Geometry: final body of the model. Coordinates: model frame, mm. Coordinates: 2 decimals unless noted, no trailing zeros. Loops run counter-clockwise (first coordinate to the right, second up) from the corner with the lowest first, then second, coordinate; pieces in that order, holes last. Notation, with made-up numbers: (55.5, 10.25) - (114.5, 10.25) arc R35 ccw to (114.5, 45.25) - close; hole circle Ø1 at (-14.5, 81). An arc over 180 degrees is marked (long way). Write each question's results on one line, items separated by ' | '. Start each with the question number.
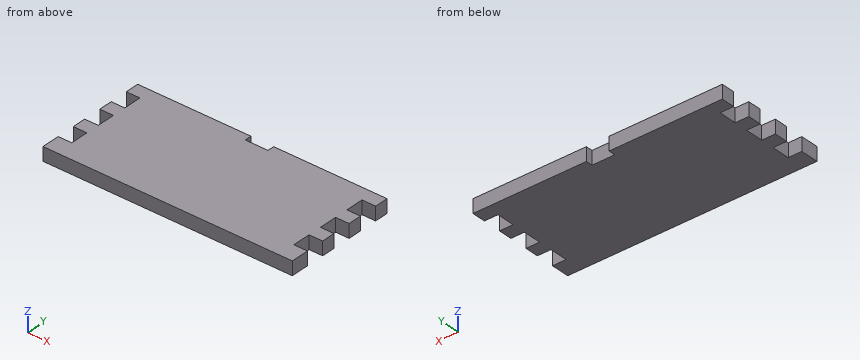
from build123d import *

# Parameters (mm, degrees)
SKETCH1_W           = 55
SKETCH1_H           = 25
BOSS_EXTRUDE1_DEPTH = 3
SKETCH2_W           = 5
SKETCH2_H           = 1.5
CUT_EXTRUDE1_DEPTH  = 3
SKETCH3_W           = 3
SKETCH3_H           = 4
CUT_EXTRUDE2_DEPTH  = 3
SKETCH4_W           = 3
SKETCH4_H           = 4
CUT_EXTRUDE3_DEPTH  = 3


with BuildPart() as part:
    # Sketch1 → Boss-Extrude1 (new body)
    with BuildSketch(Plane.XY):
        Rectangle(SKETCH1_W, SKETCH1_H)
    extrude(amount=BOSS_EXTRUDE1_DEPTH)

    # Sketch2 → Cut-Extrude1 (cut)
    with BuildSketch(Plane.XY.offset(3)):
        with Locations((0, 11.75)):
            Rectangle(SKETCH2_W, SKETCH2_H)
    extrude(amount=-CUT_EXTRUDE1_DEPTH, mode=Mode.SUBTRACT)

    # Sketch3 → Cut-Extrude2 (cut)
    with BuildSketch(Plane.XY.offset(3)):
        with Locations((-26, 7.5)):
            Rectangle(SKETCH3_W, SKETCH3_H)
        with Locations((-26, 0.5)):
            Rectangle(SKETCH3_W, SKETCH3_H)
        with Locations((-26, -6.5)):
            Rectangle(SKETCH3_W, SKETCH3_H)
    extrude(amount=-CUT_EXTRUDE2_DEPTH, mode=Mode.SUBTRACT)

    # Sketch4 → Cut-Extrude3 (cut)
    with BuildSketch(Plane.XY.offset(3)):
        with Locations((26, 7.5)):
            Rectangle(SKETCH4_W, SKETCH4_H)
        with Locations((26, 0.5)):
            Rectangle(SKETCH4_W, SKETCH4_H)
        with Locations((26, -6.5)):
            Rectangle(SKETCH4_W, SKETCH4_H)
    extrude(amount=-CUT_EXTRUDE3_DEPTH, mode=Mode.SUBTRACT)


solid = part.part
1) Pin query (flat end, axial travel): pin 1 Ø0.9 at (y, z) = (8, 1.5) entering from -X; pin 2 Ø1.5 at (y, z) = (7, 2) entering from +X. Return the tip coordinate at first contact, or that it passes through.
2) Material intervals for line 1 (X direction, y = -4.75, z = 2.8); line 2 (Y direction, x = -1, z = 1.55), sorted ascending. Write a range as [from, to].
3) Section query B-B on y = 2. Output: boundary loops of the cut face in (x, z), and give its area (3 significant figures).
Returned:
1) pin 1: stops at x = -24.5 | pin 2: stops at x = 24.5
2) line 1: x = [-24.5, 24.5] | line 2: y = [-12.5, 11]
3) outline: (-24.5, 0) - (24.5, 0) - (24.5, 3) - (-24.5, 3) - close | area: 147 mm²
